Source: CAD feature listing. Evaluate the final solid. Frame: model axes, mm. A direction names the side the tool comes from. Give positions to 0.01 mm unless a question says otherwise; leave off trailing zeros. Loops run counter-clockwise (first coordinate to the right, second up) from the corner with the lowest first, then second, coordinate; pieces in that order, holes last.
from build123d import *

# Parameters (mm, degrees)
F0_R     = 10
F0_R_2   = 9.5
F0_R_3   = 1
F1_DEPTH = 2
F2_DEPTH = 12
F3_R     = 10
F3_R_2   = 9.5
F3_R_3   = 1
F4_DEPTH = 2
F5_DEPTH = 8
F6_DEPTH = 20
F7_DEPTH = 1


with BuildPart() as f1:
    # F0 (on Front) → F1 (new body)
    with BuildSketch(Plane.XZ):
        Circle(F0_R)
        Circle(F0_R_2, mode=Mode.SUBTRACT)
        Circle(F0_R_2)
        with BuildLine():
            ThreePointArc((4.3301270189, 2.5), (4.8296291314, 1.2940952255), (5, 0))
            ThreePointArc((5, 0), (4.8296291314, -1.2940952255), (4.3301270189, -2.5))
            ThreePointArc((4.3301270189, -2.5), (2.5, -4.3301270189), (0, -5))
            ThreePointArc((0, -5), (-2.5, -4.3301270189), (-4.3301270189, -2.5))
            ThreePointArc((-4.3301270189, -2.5), (-5, 0), (-4.3301270189, 2.5))
            ThreePointArc((-4.3301270189, 2.5), (-2.5, 4.3301270189), (0, 5))
            ThreePointArc((0, 5), (2.5, 4.3301270189), (4.3301270189, 2.5))
        make_face(mode=Mode.SUBTRACT)
        with BuildLine():
            Line((0, 5), (4.3301270189, 2.5))
            ThreePointArc((4.3301270189, 2.5), (2.5, 4.3301270189), (0, 5))
        make_face()
        with BuildLine():
            Line((-4.3301270189, 2.5), (0, 5))
            ThreePointArc((0, 5), (-2.5, 4.3301270189), (-4.3301270189, 2.5))
        make_face()
        with BuildLine():
            Line((-4.3301270189, -2.5), (-4.3301270189, 2.5))
            ThreePointArc((-4.3301270189, 2.5), (-5, 0), (-4.3301270189, -2.5))
        make_face()
        with BuildLine():
            ThreePointArc((-4.3301270189, -2.5), (-2.5, -4.3301270189), (0, -5))
            Line((0, -5), (-4.3301270189, -2.5))
        make_face()
        with BuildLine():
            ThreePointArc((0, -5), (2.5, -4.3301270189), (4.3301270189, -2.5))
            Line((4.3301270189, -2.5), (0, -5))
        make_face()
        Polygon((4.3301270189, -2.5), (4.3301270189, 2.5), (0, 5), (-4.3301270189, 2.5), (-4.3301270189, -2.5), (0, -5), align=None)
        Circle(F0_R_3, mode=Mode.SUBTRACT)
        with BuildLine():
            ThreePointArc((4.3301270189, -2.5), (4.8296291314, -1.2940952255), (5, 0))
            ThreePointArc((5, 0), (4.8296291314, 1.2940952255), (4.3301270189, 2.5))
            Line((4.3301270189, 2.5), (4.3301270189, -2.5))
        make_face()
    extrude(amount=F1_DEPTH)

    # F0 (on Front) → F2 (join)
    with BuildSketch(Plane.XZ):
        Circle(F0_R_2)
        with BuildLine():
            ThreePointArc((4.3301270189, 2.5), (4.8296291314, 1.2940952255), (5, 0))
            ThreePointArc((5, 0), (4.8296291314, -1.2940952255), (4.3301270189, -2.5))
            ThreePointArc((4.3301270189, -2.5), (2.5, -4.3301270189), (0, -5))
            ThreePointArc((0, -5), (-2.5, -4.3301270189), (-4.3301270189, -2.5))
            ThreePointArc((-4.3301270189, -2.5), (-5, 0), (-4.3301270189, 2.5))
            ThreePointArc((-4.3301270189, 2.5), (-2.5, 4.3301270189), (0, 5))
            ThreePointArc((0, 5), (2.5, 4.3301270189), (4.3301270189, 2.5))
        make_face(mode=Mode.SUBTRACT)
        Polygon((4.3301270189, -2.5), (4.3301270189, 2.5), (0, 5), (-4.3301270189, 2.5), (-4.3301270189, -2.5), (0, -5), align=None)
        Circle(F0_R_3, mode=Mode.SUBTRACT)
        with BuildLine():
            Line((-4.3301270189, 2.5), (0, 5))
            ThreePointArc((0, 5), (-2.5, 4.3301270189), (-4.3301270189, 2.5))
        make_face()
        with BuildLine():
            Line((0, 5), (4.3301270189, 2.5))
            ThreePointArc((4.3301270189, 2.5), (2.5, 4.3301270189), (0, 5))
        make_face()
        with BuildLine():
            ThreePointArc((4.3301270189, -2.5), (4.8296291314, -1.2940952255), (5, 0))
            ThreePointArc((5, 0), (4.8296291314, 1.2940952255), (4.3301270189, 2.5))
            Line((4.3301270189, 2.5), (4.3301270189, -2.5))
        make_face()
        with BuildLine():
            Line((-4.3301270189, -2.5), (-4.3301270189, 2.5))
            ThreePointArc((-4.3301270189, 2.5), (-5, 0), (-4.3301270189, -2.5))
        make_face()
        with BuildLine():
            ThreePointArc((-4.3301270189, -2.5), (-2.5, -4.3301270189), (0, -5))
            Line((0, -5), (-4.3301270189, -2.5))
        make_face()
        with BuildLine():
            ThreePointArc((0, -5), (2.5, -4.3301270189), (4.3301270189, -2.5))
            Line((4.3301270189, -2.5), (0, -5))
        make_face()
    extrude(amount=F2_DEPTH)



with BuildPart() as f4:
    # F3 (on face) → F4 (new body)
    with BuildSketch(Plane.XZ.offset(12)):
        Circle(F3_R)
        Circle(F3_R_2, mode=Mode.SUBTRACT)
        Circle(F3_R_2)
        with BuildLine():
            ThreePointArc((4.3301270189, 2.5), (4.8296291314, 1.2940952255), (5, 0))
            ThreePointArc((5, 0), (4.8296291314, -1.2940952255), (4.3301270189, -2.5))
            ThreePointArc((4.3301270189, -2.5), (2.5, -4.3301270189), (0, -5))
            ThreePointArc((0, -5), (-2.5, -4.3301270189), (-4.3301270189, -2.5))
            ThreePointArc((-4.3301270189, -2.5), (-5, 0), (-4.3301270189, 2.5))
            ThreePointArc((-4.3301270189, 2.5), (-2.5, 4.3301270189), (0, 5))
            ThreePointArc((0, 5), (2.5, 4.3301270189), (4.3301270189, 2.5))
        make_face(mode=Mode.SUBTRACT)
        with BuildLine():
            Line((-4.3301270189, 2.5), (0, 5))
            ThreePointArc((0, 5), (-2.5, 4.3301270189), (-4.3301270189, 2.5))
        make_face()
        with BuildLine():
            Line((-4.3301270189, -2.5), (-4.3301270189, 2.5))
            ThreePointArc((-4.3301270189, 2.5), (-5, 0), (-4.3301270189, -2.5))
        make_face()
        with BuildLine():
            Line((0, 5), (4.3301270189, 2.5))
            ThreePointArc((4.3301270189, 2.5), (2.5, 4.3301270189), (0, 5))
        make_face()
        Polygon((4.3301270189, -2.5), (4.3301270189, 2.5), (0, 5), (-4.3301270189, 2.5), (-4.3301270189, -2.5), (0, -5), align=None)
        Circle(F3_R_3, mode=Mode.SUBTRACT)
        with BuildLine():
            ThreePointArc((4.3301270189, -2.5), (4.8296291314, -1.2940952255), (5, 0))
            ThreePointArc((5, 0), (4.8296291314, 1.2940952255), (4.3301270189, 2.5))
            Line((4.3301270189, 2.5), (4.3301270189, -2.5))
        make_face()
        with BuildLine():
            ThreePointArc((0, -5), (2.5, -4.3301270189), (4.3301270189, -2.5))
            Line((4.3301270189, -2.5), (0, -5))
        make_face()
        with BuildLine():
            ThreePointArc((-4.3301270189, -2.5), (-2.5, -4.3301270189), (0, -5))
            Line((0, -5), (-4.3301270189, -2.5))
        make_face()
    extrude(amount=F4_DEPTH)


with BuildPart() as f1_1:
    add(f1.part)

    add(f4.part)  # F5 merges F4
    # F3 (on face) → F5 (join)
    with BuildSketch(Plane.XZ.offset(12)):
        Polygon((4.3301270189, -2.5), (4.3301270189, 2.5), (0, 5), (-4.3301270189, 2.5), (-4.3301270189, -2.5), (0, -5), align=None)
        Circle(F3_R_3, mode=Mode.SUBTRACT)
    extrude(amount=F5_DEPTH)

    # F3 (on face) → F6 (cut)
    with BuildSketch(Plane.XZ.offset(12)):
        Circle(F3_R_3)
    extrude(amount=F6_DEPTH, mode=Mode.SUBTRACT)

    # F3 (on face) → F7 (join)
    with BuildSketch(Plane.XZ.offset(12)):
        Circle(F3_R)
        Circle(F3_R_2, mode=Mode.SUBTRACT)
    extrude(amount=-F7_DEPTH)


solid = f1_1.part
1) Reachability of faces 1 (the flat face through (9, -2, -4)), 2 (the flat face through (2.13, -16.96, -3.77)), 3 (the flat face through (-5, -14, 0)) from +Z, -Z, +X, -X, +Y, -Y: full face, straight path, thin tool, end or side. Return the list, or none.
Checks:
face 1: none
face 2: -Z, +X, -Y
face 3: -Y
2) Ray query, probe 1 along Z at (x, y) = (0, -13); probe 2 along Y at (x, z) = (1.25, -6.5); probe 3 along Z at (x, y) = (0, -10). Return the intervals inside material, ascending.
Checks:
probe 1: z = -10 to -1, 1 to 10
probe 2: y = -14 to 0
probe 3: z = -9.5 to -1, 1 to 9.5
3) Cut plane B-B (y = -18.5). Return loops of the section in (x, z), and give its area (3 significant figures).
Checks:
outline: (-4.33, -2.5) - (0, -5) - (4.33, -2.5) - (4.33, 2.5) - (0, 5) - (-4.33, 2.5) - close; hole circle Ø2 at (0, 0)
area: 61.8 mm2
4) Pull-direction query (Z, two-part tool) for faces 4 (the flat face through (-2.2, -16.96, -3.73)), 5 (the cylindrical face through (0, -10, -1)), 6 (the flat face through (-2.13, -16.96, 3.77)); classes: released by +Z, released by -Z, zero draft, split by the parting line, or undercut.
Checks:
face 4: released by -Z
face 5: undercut
face 6: released by +Z
5) Cut plane D-D (x = -7.5). Return loops of the section in (y, z).
Checks:
outline: (-14, -6.61) - (-11, -6.61) - (-11, -5.83) - (-2, -5.83) - (-2, -6.61) - (0, -6.61) - (0, 6.61) - (-2, 6.61) - (-2, 5.83) - (-11, 5.83) - (-11, 6.61) - (-14, 6.61) - close
6) Cut plane A-A (z = 0). Return loops of the section in (x, y), and give its area (3 significant figures).
Checks:
outline: (-10, -14) - (-4.33, -14) - (-4.33, -20) - (-1, -20) - (-1, 0) - (-10, 0) - (-10, -2) - (-9.5, -2) - (-9.5, -11) - (-10, -11) - close; (1, -20) - (4.33, -20) - (4.33, -14) - (10, -14) - (10, -11) - (9.5, -11) - (9.5, -2) - (10, -2) - (10, 0) - (1, 0) - close
area: 283 mm2
7) Cut plane C-C (x = -0.5). Return loops of the section in (y, z).
Checks:
outline: (-20, -4.71) - (-14, -4.71) - (-14, -9.99) - (-11, -9.99) - (-11, -9.49) - (-2, -9.49) - (-2, -9.99) - (0, -9.99) - (0, -0.87) - (-20, -0.87) - close; (-20, 0.87) - (0, 0.87) - (0, 9.99) - (-2, 9.99) - (-2, 9.49) - (-11, 9.49) - (-11, 9.99) - (-14, 9.99) - (-14, 4.71) - (-20, 4.71) - close
8) Contact query for flat-ended pins moving along their axis: P1, Ø1, axis at y = -8.5, z = -1.5, coming from the +X side; P2, Ø6, axis at y = -7.5, z = 7, coming from the +X side; P3, Ø5, axis at x = 6.5, y = -2.5, coming from the +Z side. Output: stop coordinate, or through.
Checks:
P1: stops at x = 9.45
P2: stops at x = 8.62
P3: stops at z = 9.14
